Input: part model. Units: mm. Frame: model coordinates. A direction names the side the tool comes from. Round coordinates to 2 decimals unless told otherwise and drop trailing zeros. Loops run counter-clockwise (first coordinate to the right, second up) from the corner with the lowest first, then second, coordinate; pieces in that order, holes last. Notation, with made-up numbers: (-13, -21.75) - (-9, -21.75) arc R22 ccw to (-9, 13.25) - close; hole circle Ø4 at (86, -20.75). An arc over 180 degrees is marked (long way). One line per question, with ' | ' between items. Start each with the question number.
from build123d import *

# Parameters (mm, degrees)
TAP_DRILL_FOR_M3_HELICOIL1_D = 3.15
SKETCH10_W                   = 44.45
SKETCH10_H                   = 44.45
SKETCH10_W_2                 = 31.75
SKETCH10_H_2                 = 31.75
CUT_EXTRUDE2_DEPTH           = 39.1000001
SKETCH11_R                   = 9.525
CUT_EXTRUDE3_DEPTH           = 25.4


with BuildPart() as part:
    # Sketch1 → Revolve1 (revolve)
    with BuildSketch(Plane(origin=(0, 0, 0), x_dir=(1, 0, 0), z_dir=(0, 1, 0))):
        Polygon((0, 0), (0, 19.05), (38.1, 19.05), (38.1, 9.525), (38.1, 0), align=None)
    revolve(axis=Axis((0, 0, 0), (1, 0, 0)))

    # Tap Drill for M3 Helicoil1 (through all)
    with Locations(Plane(origin=(8.941446853, 14.626722755, 12.204977732), x_dir=(0, -0.640681246, 0.767806969), z_dir=(0, 0.767806969, 0.640681246))):
        with Locations((0, 0)):
            Hole(TAP_DRILL_FOR_M3_HELICOIL1_D / 2)

    # Sketch10 → Cut-Extrude2 (cut, through all)
    with BuildSketch(Plane.ZY):
        Rectangle(SKETCH10_W, SKETCH10_H)
        Rectangle(SKETCH10_W_2, SKETCH10_H_2, mode=Mode.SUBTRACT)
    extrude(amount=-CUT_EXTRUDE2_DEPTH, mode=Mode.SUBTRACT)

    # Sketch11 → Cut-Extrude3 (cut)
    with BuildSketch(Plane.ZY):
        Circle(SKETCH11_R)
    extrude(amount=-CUT_EXTRUDE3_DEPTH, mode=Mode.SUBTRACT)


solid = part.part
(1) Pull-direction query (Z, two-part tool) for faces 1 (the face through (19.32, 13.43, -13.51)), 2 (the face through (0, -7, -7)), 3 (the face through (25.4, 0, 0)); classes: released by +Z, released by -Z, zero draft, split by the parting line, or undercut.
(2) Reachability of faces 4 (the face through (9.41, -10.01, -10.31)), 5 (the face through (12.522, -5.796, -7.559)) from +Z, -Z, +X, -X, +Y, -Y: full face, straight path, thin tool, end or side. Return the list, or none.
(3) Section B-B, the plane y = 0. Output: boundary loops of the cut face in (x, z) (3 decimals), plus the area to 3 significant figures.
(4) Section A-A, the plane x = 22. Output: boundary loops of the cut face in (y, z) (3 decimals), plus the area to 3 significant figures.
(5) Line query: line 1 along Y through (x, z) = (6, 0) (3 decimals); line 2 along X through (y, z) = (-2.5, 7.5); line 3 along Z through (x, y) = (3, 3.5) (3 decimals). Output: solid intervals per line, ascending. Write a range as from..to.
(6) Pin query (flat end, axial travel): P1, Ø3, axis at x = 22.5, z = 11, coming from the +Y side (3 decimals). Return the tip coordinate at first contact, or that it passes through.
Derived:
1) face 1: released by -Z | face 2: zero draft | face 3: undercut
2) face 4: none | face 5: -X
3) outline: (0, -15.875) - (38.1, -15.875) - (38.1, 15.875) - (0, 15.875) - (0, 9.525) - (25.4, 9.525) - (25.4, -9.525) - (0, -9.525) - close | area: 726 mm²
4) outline: (-15.875, -10.53) arc R19.05 ccw to (-10.53, -15.875) - (10.53, -15.875) arc R19.05 ccw to (15.875, -10.53) - (15.875, 10.53) arc R19.05 ccw to (10.53, 15.875) - (-10.53, 15.875) arc R19.05 ccw to (-15.875, 10.53) - close; hole circle Ø19.05 at (0, 0) | area: 674 mm²
5) line 1: y = -15.875..-9.525, 9.525..15.875 | line 2: x = 25.4..38.1 | line 3: z = -15.875..-8.859, 8.859..15.875
6) P1: stops at y = 15.875
